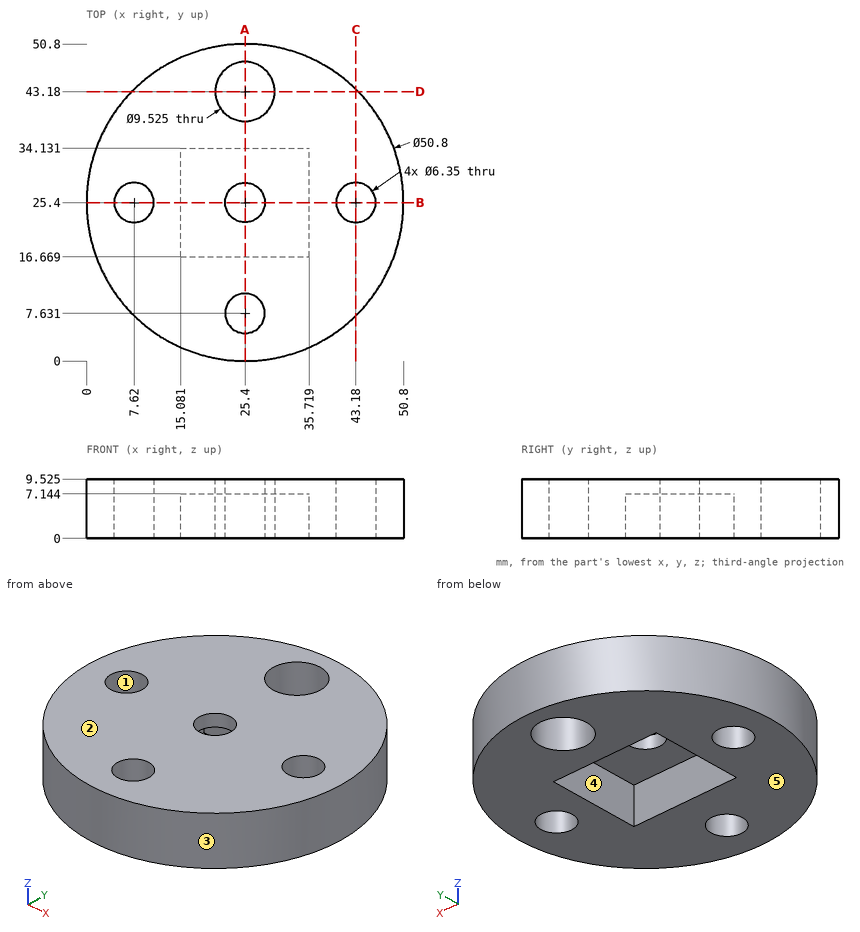
Geometry check sheet. Reference: drawing and pictorial views, mm from the part's lowest x, y, z. A direction names the side the tool comes from. Round coordinates to 2 decimals unless told otherwise and drop trailing zeros. Write each loop counter-clockwise with the first axis right and the second up, starting at its lowest first coordinate (ties: lowest second). Pieces come first, ordered by that corner, then holes.
Item 1: Section check A-A (x = 25.4). Record the boundary of the cut face in (y, z) (1 decimal).
Determined:
outline: (0, 0) - (4.5, 0) - (4.5, 9.5) - (0, 9.5) - close; (10.8, 0) - (16.7, 0) - (16.7, 7.1) - (22.2, 7.1) - (22.2, 9.5) - (10.8, 9.5) - close; (28.6, 7.1) - (34.1, 7.1) - (34.1, 0) - (38.4, 0) - (38.4, 9.5) - (28.6, 9.5) - close; (47.9, 0) - (50.8, 0) - (50.8, 9.5) - (47.9, 9.5) - close
Item 2: Section check D-D (y = 43.18). Record the boundary of the cut face in (x, z) (1 decimal).
Determined:
outline: (7.3, 0) - (20.6, 0) - (20.6, 9.5) - (7.3, 9.5) - close; (30.2, 0) - (43.5, 0) - (43.5, 9.5) - (30.2, 9.5) - close
Item 3: Material ranges on line 1 along Y through (x, z) = (25.4, 8.65) (1 decimal); line 2 along Y through (x, z) = (25.4, 6.75); line 3 along Y through (x, z) = (21.5, 4) (1 decimal), recorded low to high.
Determined:
line 1: y = 0 to 4.5, 10.8 to 22.2, 28.6 to 38.4, 47.9 to 50.8
line 2: y = 0 to 4.46, 10.81 to 16.67, 34.13 to 38.42, 47.94 to 50.8
line 3: y = 0.3 to 16.7, 34.1 to 40.4, 45.9 to 50.5
Item 4: Go/stop test with flat-tipped pins: pin 1 Ø2 at (x, z) = (12.5, 6.5) entering from -Y; pin 2 Ø5 at (x, y) = (25.4, 25.4) entering from +Z; pin 3 Ø3 at (y, z) = (18, 4.5) entering from -X (1 decimal); pin 4 Ø8.5 at (x, y) = (25.4, 7.63) entering from +Z (3 decimals). Record where each tip stops, or that it passes through.
Determined:
pin 1: stops at y = 2.96
pin 2: passes through
pin 3: stops at x = 0.7
pin 4: stops at z = 9.525
Item 5: Mould release check, pull along Y, two halves, no side actions. Record for the marked faces 1, 2 and 3: +Y half, -Y half, draft (parallel to the pull), parting line (faces both ways), or undercut.
Determined:
face 1: undercut
face 2: draft
face 3: parting line
Item 6: Access from +Z, -Z, +X, -X, +Y, -Y to the whole of each face (thin tool, end or side, straight path). Record for the marked faces 4 and 5.
Determined:
face 4: -Z
face 5: -Z, +X, -X, +Y, -Y
Item 7: Section check C-C (x = 43.18). Record the boundary of the cut face in (y, z) (1 decimal).
Determined:
outline: (7.3, 0) - (22.2, 0) - (22.2, 9.5) - (7.3, 9.5) - close; (28.6, 0) - (43.5, 0) - (43.5, 9.5) - (28.6, 9.5) - close
Item 8: Section check B-B (y = 25.4). Record the boundary of the cut face in (x, z) (1 decimal), plus the area to 3 significant figures.
Determined:
outline: (0, 0) - (4.4, 0) - (4.4, 9.5) - (0, 9.5) - close; (10.8, 0) - (15.1, 0) - (15.1, 7.1) - (22.2, 7.1) - (22.2, 9.5) - (10.8, 9.5) - close; (28.6, 7.1) - (35.7, 7.1) - (35.7, 0) - (40, 0) - (40, 9.5) - (28.6, 9.5) - close; (46.4, 0) - (50.8, 0) - (50.8, 9.5) - (46.4, 9.5) - close
area: 200 mm2
